```python
from build123d import *

# Parameters (mm, degrees)
BOSS_EXTRUDE1_DEPTH = 5.5
SKETCH2_R           = 20
BOSS_EXTRUDE2_DEPTH = 2.5
CUT_EXTRUDE1_DEPTH  = 8
SKETCH4_W           = 3
SKETCH4_H           = 3
CUT_EXTRUDE2_DEPTH  = 10
SKETCH5_R           = 5
BOSS_EXTRUDE3_DEPTH = 140


with BuildPart() as part:
    # Sketch1 → Boss-Extrude1 (new body)
    with BuildSketch(Plane(origin=(0, 0, 0), x_dir=(1, 0, 0), z_dir=(0, 1, 0))):
        with BuildLine():
            ThreePointArc((-1.9, -2.05669638), (-2.8, 0), (-1.9, 2.05669638))
            Line((-1.9, 2.05669638), (-1.9, 5.532856405))
            ThreePointArc((-1.9, 5.532856405), (-5.85, 0), (-1.9, -5.532856405))
            Line((-1.9, -5.532856405), (-1.9, -2.05669638))
        make_face()
        with BuildLine():
            ThreePointArc((-1.9, 2.05669638), (0, 2.8), (1.9, 2.05669638))
            Line((1.9, 2.05669638), (1.9, 5.532856405))
            ThreePointArc((1.9, 5.532856405), (0, 5.85), (-1.9, 5.532856405))
            Line((-1.9, 5.532856405), (-1.9, 2.05669638))
        make_face()
        with BuildLine():
            Line((1.9, 5.532856405), (1.9, 2.05669638))
            ThreePointArc((1.9, 2.05669638), (2.565151068, 1.122497216), (2.8, 0))
            ThreePointArc((2.8, 0), (2.565151068, -1.122497216), (1.9, -2.05669638))
            Line((1.9, -2.05669638), (1.9, -5.532856405))
            ThreePointArc((1.9, -5.532856405), (4.761171074, -3.399080758), (5.85, 0))
            ThreePointArc((5.85, 0), (4.761171074, 3.399080758), (1.9, 5.532856405))
        make_face()
        with BuildLine():
            Line((1.9, -5.532856405), (1.9, -2.05669638))
            ThreePointArc((1.9, -2.05669638), (0, -2.8), (-1.9, -2.05669638))
            Line((-1.9, -2.05669638), (-1.9, -5.532856405))
            ThreePointArc((-1.9, -5.532856405), (0, -5.85), (1.9, -5.532856405))
        make_face()
        with BuildLine():
            Line((-1.9, -2.05669638), (-1.9, 2.05669638))
            ThreePointArc((-1.9, 2.05669638), (-2.8, 0), (-1.9, -2.05669638))
        make_face()
        with BuildLine():
            ThreePointArc((2.8, 0), (2.565151068, 1.122497216), (1.9, 2.05669638))
            Line((1.9, 2.05669638), (1.9, -2.05669638))
            ThreePointArc((1.9, -2.05669638), (2.565151068, -1.122497216), (2.8, 0))
        make_face()
    boss_extrude1 = extrude(amount=BOSS_EXTRUDE1_DEPTH)

    # Sketch2 → Boss-Extrude2 (add)
    with BuildSketch(Plane(origin=(0, 5.5, 0), x_dir=(1, 0, 0), z_dir=(0, 1, 0))):
        with Locations(Location((0, 0, 0), (0, 0, 270))):
            Circle(SKETCH2_R)
    boss_extrude2 = extrude(amount=-BOSS_EXTRUDE2_DEPTH)

    # Sketch3 → Cut-Extrude1 (cut)
    with BuildSketch(Plane.XZ.offset(-3)):
        with BuildLine():
            Line((-1.9, 2.05669638), (-1.9, -2.05669638))
            ThreePointArc((-1.9, -2.05669638), (0, -2.8), (1.9, -2.05669638))
            Line((1.9, -2.05669638), (1.9, 2.05669638))
            ThreePointArc((1.9, 2.05669638), (0, 2.8), (-1.9, 2.05669638))
        make_face()
    extrude(amount=-CUT_EXTRUDE1_DEPTH, mode=Mode.SUBTRACT)

    # Sketch4 → Cut-Extrude2 (cut)
    with BuildSketch(Plane(origin=(0, 5.5, 0), x_dir=(1, 0, 0), z_dir=(0, 1, 0))):
        with Locations((0, 19.8)):
            Rectangle(SKETCH4_W, SKETCH4_H)
        with Locations((20, 0)):
            Rectangle(SKETCH4_W, SKETCH4_H)
        with Locations((0, -20)):
            Rectangle(SKETCH4_W, SKETCH4_H)
        with Locations((-20, 0)):
            Rectangle(SKETCH4_W, SKETCH4_H)
    cut_extrude2 = extrude(amount=-CUT_EXTRUDE2_DEPTH, mode=Mode.SUBTRACT)

    # Sketch5 → Boss-Extrude3 (add)
    with BuildSketch(Plane(origin=(0, 5.5, 0), x_dir=(1, 0, 0), z_dir=(0, 1, 0))):
        with Locations(Location((0, 0, 0), (0, 0, 270))):
            Circle(SKETCH5_R)
    extrude(amount=BOSS_EXTRUDE3_DEPTH)

    # Mirror1: Boss-Extrude2 across plane
    add(boss_extrude2.mirror(Plane.ZX.offset(75.5)))

    # Mirror2: Boss-Extrude1, Cut-Extrude2 across plane
    add(boss_extrude1.mirror(Plane.ZX.offset(75.5)))
    add(cut_extrude2.mirror(Plane.ZX.offset(75.5)), mode=Mode.SUBTRACT)


solid = part.part
```
Read the model definition and answer for the solid it produces. Units are mm, in the model's axes. A direction names the side the tool comes from. Coordinates: 2 decimals unless noted, no trailing zeros. Loops run counter-clockwise (first coordinate to the right, second up) from the corner with the lowest first, then second, coordinate; pieces in that order, holes last. Notation, with made-up numbers: (-23.5, 50.5) - (14.5, 50.5) arc R20 ccw to (14.5, 57.5) - close; hole circle Ø6 at (2, 22.25). An arc over 180 degrees is marked (long way). Answer in a Markdown table with one row per item.
1. Which of the six approach directions +Z, -Z, +X, -X, +Y, -Y give full straight-line access (tool end or side, diameter ignored) to faces 4 (the face through (-4.88, 74.52, -1.08)), 5 (the face through (0, 147, -18.3)), 6 (the face through (-18.5, 147, 0))?
Conclusion:
| item | result |
|---|---|
| face 4 | none |
| face 5 | -Z, +Y, -Y |
| face 6 | -X, +Y, -Y |
2. Find section A-A, the plane x = -10. Write down the section's boundary in (y, z).
Conclusion:
| item | result |
|---|---|
| outline | (3, -17.32) - (5.5, -17.32) - (5.5, 17.32) - (3, 17.32) - close; (145.5, -17.32) - (148, -17.32) - (148, 17.32) - (145.5, 17.32) - close |
3. Determine the mould class of faces 1 (the face through (0, 149.5, -2.8)), 2 (the face through (-4, 145.5, 4)), 3 (the face through (-14.282, 146.732, 14.001)) for opening direction X: +X half, -X half, draft (parallel to the pull), parting line (faces both ways), or undercut.
Conclusion:
| item | result |
|---|---|
| face 1 | undercut |
| face 2 | draft |
| face 3 | -X half |
4. Given pin 1 (5 mm diameter, centred on y = 126, z = 6.5, fed in from -X); pin 2 (0.8 mm diameter, centred on x = 0.5, y = 147, fed in from -Z); pin 3 (1.6 mm diameter, centred on x = 19, y = 4.5, fed in from -Z), each flat-ended and moving along its own axis, determine where each tip first touches the part or whether it passes through.
Conclusion:
| item | result |
|---|---|
| pin 1 | stops at x = -3 |
| pin 2 | stops at z = -18.3 |
| pin 3 | stops at z = -8.29 |
5. Find section D-D, the plane y = 13. Write down the section's boundary in (x, z).
Conclusion:
| item | result |
|---|---|
| outline | circle Ø10 at (0, 0) |
6. Find section C-C, the plane x = 13.5. Write down the section's boundary in (y, z), then the cut area to 3 significant figures.
Conclusion:
| item | result |
|---|---|
| outline | (3, -14.76) - (5.5, -14.76) - (5.5, 14.76) - (3, 14.76) - close; (145.5, -14.76) - (148, -14.76) - (148, 14.76) - (145.5, 14.76) - close |
| area | 148 mm² |
7. Straight lines are drawn through the part: line 1 (Y direction, x = -3, z = -9); line 2 (X direction, y = 138.5, z = -2.5); line 3 (X direction, y = 12, z = -1). For each, find the intervals that lie inside material, in ascending order.
Conclusion:
| item | result |
|---|---|
| line 1 | y = 3 to 5.5, 145.5 to 148 |
| line 2 | x = -4.33 to 4.33 |
| line 3 | x = -4.9 to 4.9 |
8. Find section B-B, the plane x = 0. Write down the section's boundary in (y, z), then the cut area to 3 significant figures.
Conclusion:
| item | result |
|---|---|
| outline | (0, -5.85) - (3, -5.85) - (3, -18.3) - (5.5, -18.3) - (5.5, -5) - (145.5, -5) - (145.5, -18.3) - (148, -18.3) - (148, -5.85) - (151, -5.85) - (151, -2.8) - (148, -2.8) - (148, 2.8) - (151, 2.8) - (151, 5.85) - (148, 5.85) - (148, 18.5) - (145.5, 18.5) - (145.5, 5) - (5.5, 5) - (5.5, 18.5) - (3, 18.5) - (3, 5.85) - (0, 5.85) - (0, 2.8) - (5.5, 2.8) - (5.5, -2.8) - (0, -2.8) - close |
| area | 1,610 mm² |
